Check sheet for the modelled part. Datum: model origin and axes. Units: mm. Give positions to 0.01 mm unless a question says otherwise; leave off trailing zeros. Loops run counter-clockwise (first coordinate to the right, second up) from the corner with the lowest first, then second, coordinate; pieces in that order, holes last. Notation, with made-up numbers: (57.5, 62.25) - (85.5, 62.25) arc R17 cw to (85.5, 67.25) - close; hole circle Ø7 at (42, -32). An arc over 180 degrees is marked (long way). Use CSV: the item, a comma, the result in double quotes.
from build123d import *

# Parameters (mm, degrees)
F1_W     = 76.560207
F1_H     = 76.388307
F2_DEPTH = 76.2
F3_R     = 35.56
F0_D     = 5.08


with BuildPart() as f2:
    # F1 (on Top) → F2 (new body)
    with BuildSketch(Plane.XY):
        with Locations((38.280103, 38.194153)):
            Rectangle(F1_W, F1_H)
    extrude(amount=F2_DEPTH)

    # F3
    f3_edges = [f2.edges().sort_by_distance(p)[0] for p in [
        (76.560207, 76.388307, 38.1),
        (0, 76.388307, 38.1),
        (38.280103, 76.388307, 0),
        (38.280103, 76.388307, 76.2),
        (38.280103, 0, 76.2),
        (0, 38.194153, 76.2),
        (76.560207, 0, 38.1),
        (0, 38.194153, 0),
        (0, 0, 38.1),
        (38.280103, 0, 0),
        (76.560207, 38.194153, 0),
        (76.560207, 38.194153, 76.2),
    ]]
    fillet(f3_edges, radius=F3_R)

    # F0 (through all)
    with Locations(Plane.XY.offset(76.2)):
        with Locations((38.280103, 38.194153)):
            Hole(F0_D / 2)


solid = f2.part
1. Sectioned sample at C-C, the plane x = 16.5. Record the boundary of the cut face in (y, z), and give its area (3 significant figures).
Completed:
outline,"(5.54, 35.56) arc R30.02 ccw to (35.56, 5.54) - (40.83, 5.54) arc R30.02 ccw to (70.85, 35.56) - (70.85, 40.64) arc R30.02 ccw to (40.83, 70.66) - (35.56, 70.66) arc R30.02 ccw to (5.54, 40.64) - close"
area,"3,480 mm²"
2. Sectioned sample at D-D, the plane z = 68. Record the boundary of the cut face in (x, y), and give its area (3 significant figures).
Completed:
outline,"(12.85, 35.56) arc R22.71 ccw to (35.56, 12.85) - (41, 12.85) arc R22.71 ccw to (63.71, 35.56) - (63.71, 40.83) arc R22.71 ccw to (41, 63.54) - (35.56, 63.54) arc R22.71 ccw to (12.85, 40.83) - close; hole circle Ø5.08 at (38.28, 38.19)"
area,"2,120 mm²"
3. Scan lines: line 1 along X through (y, z) = (39.5, 70.5); line 2 along Y through (x, z) = (10.5, 59); line 3 along X through (y, z) = (25, 5). Record each from-to range of solid material in increasing order.
Completed:
line 1,"x = 16.25 to 36.1, 40.46 to 60.31"
line 2,"y = 18.26 to 58.13"
line 3,"x = 20.76 to 55.8"
4. Go/stop test with flat-tipped pins: pin 1 Ø5 at (x, y) = (54.5, 29.5) entering from -Z; pin 2 Ø1 at (x, z) = (68.5, 48.5) entering from +Y; pin 3 Ø1.5 at (y, z) = (27, 11.5) entering from +X. Record where each tip stops, or that it passes through.
Completed:
pin 1,"stops at z = 2.19"
pin 2,"stops at y = 62.62"
pin 3,"stops at x = 66.5"
5. Sectioned sample at B-B, the plane y = 66. Record the boundary of the cut face in (x, z).
Completed:
outline,"(10.44, 35.56) arc R25.12 ccw to (35.56, 10.44) - (41, 10.44) arc R25.12 ccw to (66.12, 35.56) - (66.12, 40.64) arc R25.12 ccw to (41, 65.76) - (35.56, 65.76) arc R25.12 ccw to (10.44, 40.64) - close"
6. Sectioned sample at A-A, the plane z = 42. Record the boundary of the cut face in (x, y).
Completed:
outline,"(0.03, 35.56) arc R35.53 ccw to (35.56, 0.03) - (41, 0.03) arc R35.53 ccw to (76.53, 35.56) - (76.53, 40.83) arc R35.53 ccw to (41, 76.36) - (35.56, 76.36) arc R35.53 ccw to (0.03, 40.83) - close; hole circle Ø5.08 at (38.28, 38.19)"
7. Release check for a two-part mould opening along Y. For faces 1 (the face through (10.14, 65.695, 38.136)), 2 (the face through (36.915, 40.336, 37.567)), 3 (the face through (38.318, 10.14, 10.693)) record: released by +Y, released by -Y, zero draft, split by the parting line, or undercut.
Completed:
face 1,"released by +Y"
face 2,"undercut"
face 3,"released by -Y"
